from build123d import *

# Parameters (mm, degrees)
F0_R     = 6.5928960908
F1_DEPTH = 26
F2_COUNT = 12
F3_SIZE  = 6.3


# Not quite as in the source:
# - a feature names something its author has since deleted; it is built from what else it names


with BuildPart() as f1:
    # F0 (on Front) → F1 (new body)
    with BuildSketch(Plane.XZ):
        with BuildLine():
            ThreePointArc((-5.6485408912, 26.2598637858), (-16.878445243, -20.8950842647), (26.8605, 0))
            ThreePointArc((26.8605, 0), (20.0726478905, 17.8486768953), (3.1397750014, 26.6763616933))
            ThreePointArc((3.1397750014, 26.6763616933), (-1.2715518862, 26.8303860585), (-5.6485408912, 26.2598637858))
        make_face()
        Circle(F0_R, mode=Mode.SUBTRACT)
        with BuildLine():
            ThreePointArc((-5.6485408912, 26.2598637858), (-1.2715518862, 26.8303860585), (3.1397750014, 26.6763616933))
            ThreePointArc((3.1397750014, 26.6763616933), (2.912439248, 29.1823081791), (2.258607373, 31.6121133592))
            ThreePointArc((2.258607373, 31.6121133592), (1.0476425624, 34.1233003108), (-0.5978331908, 36.3738347416))
            Line((-0.5978331908, 36.3738347416), (-1.7586341705, 34.2293752337))
            Line((-1.7586341705, 34.2293752337), (-3.1894124709, 36.2039736615))
            ThreePointArc((-3.1894124709, 36.2039736615), (-4.5270572612, 33.7579151802), (-5.3998864293, 31.1101491555))
            ThreePointArc((-5.3998864293, 31.1101491555), (-5.727107406, 28.6954080102), (-5.6485408912, 26.2598637858))
        make_face()
    extrude(amount=F1_DEPTH)

    # F2: F1 ×12 about axis
    f2_axis = Axis((0, 0, 0), (0, 1, 0))


with BuildPart() as f1_1:
    add(f1.part)
    for i in range(1, F2_COUNT):
        add(f1.part.rotate(f2_axis, i * 360 / F2_COUNT))

    # F3
    f3_edges = [f1_1.edges().sort_by_distance(p)[0] for p in [
        (-6.592896, 0, 0),
        (6.592896, -13, 0),
        (-6.592896, -26, 0),
    ]]
    chamfer(f3_edges, length=F3_SIZE)


solid = f1_1.part
Could you check a few things on this model? Use its own coordinates, in mm. A direction names the side the tool comes from. Give positions to 0.01 mm unless a question says otherwise; leave off trailing zeros. Return JSON: item names as keys, results as strings. Group by question number.
Q1. Will these pins go through, and if not, where does the flat tip stop? pin 1 Ø1 at (x, y) = (29, -8) entering from +Z; pin 2 Ø10 at (x, y) = (10, -6.5) entering from +Z; pin 3 Ø10.5 at (x, z) = (0, 0) entering from -Y; pin 4 Ø1 at (y, z) = (-18, 20) entering from +X.
Q2. Which directions (+Z, -Z, +X, -X, +Y, -Y) give clear straight access to the entire face, cutting with the end or side of a thin tool? Please do faces 5 (the face through (-5.725, -12.818, 28.73)), 6 (the face through (26.237, -12.818, -5.752)), 7 (the face through (12.99, -12.82, 31.52)), 8 (the face through (-2.92, -12.82, -29.15)).
Q3. Thinking about a two-plate mould opening in X: for faces 1 (the face through (23.78, -12.82, -17.1)), 2 (the face through (17.97, -12.82, 28.99)), 3 (the face through (-2.46, -12.82, 35.2)), 4 (the face through (-17.97, -12.82, -28.99)), which applies, pulls with the +X half, pulls with the -X half, needs draft (parallel to the pull), parting line crosses it, or undercut?
Q4. Please list where these lines run through material, in increasing order: line 1 along Z through (x, y) = (-30, -7); line 2 along X through (y, z) = (-15, 0). Write a range as [from, to].
Resolved:
{
 "1": {"pin 1": "stops at z = 20.9", "pin 2": "stops at z = 32.78", "pin 3": "passes through", "pin 4": "stops at x = 29.6"},
 "2": {"face 5": "+Y, -Y", "face 6": "+X, +Y, -Y", "face 7": "+Z, +Y, -Y", "face 8": "-Z, +Y, -Y"},
 "3": {"face 1": "undercut", "face 2": "pulls with the +X half", "face 3": "undercut", "face 4": "pulls with the -X half"},
 "4": {"line 1": "z = [-18.67, -16.02], [-5.6, 2.74], [11.22, 17.92]", "line 2": "x = [-35.65, -6.59], [6.59, 35.65]"}
}
